```python
from build123d import *

# Parameters (mm, degrees)
EXTRUSION1_DEPTH        = 110
PER_AGE1_OUTLINE_R      = 2.1
PER_AGE1_DEPTH          = 110
ENL_V_MAT_EXTRU_1_DEPTH = 300
ENL_V_MAT_EXTRU_3_DEPTH = 300
ENL_V_MAT_EXTRU_4_DEPTH = 111.905365064
ENL_V_MAT_EXTRU_7_DEPTH = 111.905365064


# Read off the part's stored shape, not the designer's step: Perçage1
with BuildPart() as part:
    # Esquisse1 → Extrusion1 (new body)
    with BuildSketch(Plane.XY):
        with BuildLine():
            Line((-10, 8), (-10, -8))
            ThreePointArc((-10, -8), (-9.414213562, -9.414213562), (-8, -10))
            Line((-8, -10), (8, -10))
            ThreePointArc((8, -10), (9.414213562, -9.414213562), (10, -8))
            Line((10, -8), (10, 8))
            ThreePointArc((10, 8), (9.414213562, 9.414213562), (8, 10))
            Line((8, 10), (-8, 10))
            ThreePointArc((-8, 10), (-9.414213562, 9.414213562), (-10, 8))
        make_face()
    extrude(amount=EXTRUSION1_DEPTH)

    # Perçage1 outline → Perçage1 (cut)
    with BuildSketch(Plane.XY):
        Circle(PER_AGE1_OUTLINE_R)
    extrude(amount=PER_AGE1_DEPTH, mode=Mode.SUBTRACT)

    # Esquisse3 → Enlèv. mat.-Extru.1 (cut)
    with BuildSketch(Plane.XY.offset(110)):
        Polygon((10, 2.5), (8.2, 2.5), (8.2, 6), (3.7, 2.5), (3.7, -2.5), (8.2, -6), (8.2, -2.5), (10, -2.5), align=None)
    extrude(amount=-ENL_V_MAT_EXTRU_1_DEPTH, mode=Mode.SUBTRACT)

    # Esquisse5 → Enlèv. mat.-Extru.3 (cut)
    with BuildSketch(Plane.XY.offset(110)):
        Polygon((-2.5, 10), (-2.5, 8.2), (-6, 8.2), (-2.5, 3.7), (2.5, 3.7), (6, 8.2), (2.5, 8.2), (2.5, 10), align=None)
    extrude(amount=-ENL_V_MAT_EXTRU_3_DEPTH, mode=Mode.SUBTRACT)

    # Esquisse6 → Enlèv. mat.-Extru.4 (cut, through all)
    with BuildSketch(Plane.XY.offset(110)):
        Polygon((-2.5, -10), (-2.5, -8.2), (-6, -8.2), (-2.5, -3.7), (2.5, -3.7), (6, -8.2), (2.5, -8.2), (2.5, -10), align=None)
    extrude(amount=-ENL_V_MAT_EXTRU_4_DEPTH, mode=Mode.SUBTRACT)

    # Esquisse4 → Enlèv. mat.-Extru.7 (cut, through all)
    with BuildSketch(Plane.XY.offset(110)):
        Polygon((-10, 2.5), (-8.2, 2.5), (-8.2, 6), (-3.7, 2.5), (-3.7, -2.5), (-8.2, -6), (-8.2, -2.5), (-10, -2.5), align=None)
    extrude(amount=-ENL_V_MAT_EXTRU_7_DEPTH, mode=Mode.SUBTRACT)


solid = part.part
```
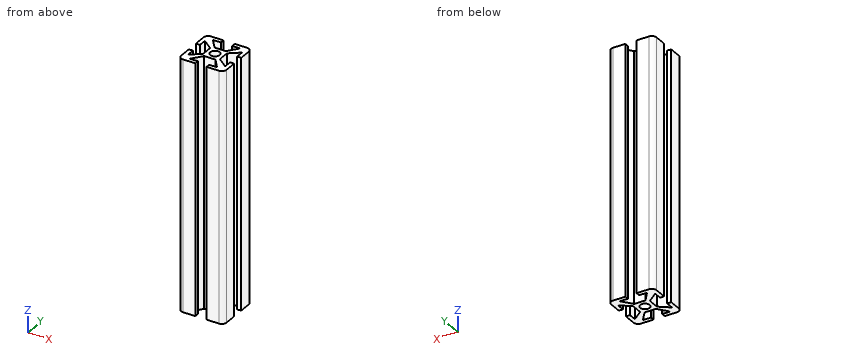
Build history of the part. All positions in model axes, mm. Give positions to 0.01 mm unless a question says otherwise; leave off trailing zeros. Loops run counter-clockwise (first coordinate to the right, second up) from the corner with the lowest first, then second, coordinate; pieces in that order, holes last. Notation, with made-up numbers: (16.5, 18) - (59.5, 18) arc R17 cw to (59.5, 37) - close; hole circle Ø3 at (79.5, 29.25). An arc over 180 degrees is marked (long way). Use a Markdown table: item, result.
(1) Drop flat-ended pins along their axis: pin 1 Ø1.4 at (x, z) = (-9, 81.5) entering from +Y; pin 2 Ø1.4 at (y, z) = (-9, 49.5) entering from +X; pin 3 Ø1.4 at (y, z) = (-9, 32.5) entering from -X. Give the stop position or say it passes through.
Taken from the geometry:
| item | result |
|---|---|
| pin 1 | y = 9.98 |
| pin 2 | x = 9.98 |
| pin 3 | x = -9.98 |
(2) Wall check: line 1 along Y through (x, z) = (0, 73.5); line 2 along Y through (x, z) = (5.25, 9.5); line 3 along Y through (x, z) = (-5.75, 96). Give the ranges that are in metal, low to high.
Taken from the geometry:
| item | result |
|---|---|
| line 1 | -3.7 to -2.1, 2.1 to 3.7 |
| line 2 | -10 to -8.2, -7.24 to -3.71, 3.71 to 7.24, 8.2 to 10 |
| line 3 | -10 to -8.2, -7.88 to -4.09, 4.09 to 7.88, 8.2 to 10 |
(3) Band-saw the part on A-A (y = 0). Give the cut face in (x, z), and give its area (3 significant figures).
Taken from the geometry:
| item | result |
|---|---|
| outline | (-3.7, 0) - (-2.1, 0) - (-2.1, 110) - (-3.7, 110) - close; (2.1, 0) - (3.7, 0) - (3.7, 110) - (2.1, 110) - close |
| area | 352 mm2 |
